Verification items for this drawing (mm, ordinates from the low corner). Give positions to 0.01 mm unless a question says otherwise; leave off trailing zeros. Loops run counter-clockwise (first coordinate to the right, second up) from the corner with the lowest first, then second, coordinate; pieces in that order, holes last. Notation, with made-up numbers: M 54,-29 L 103,-29 A9 ccw 103,-22 Z; hole C 72,-16 d6. An arc over 180 degrees is marked long. Put each result on its own line as item: value. Start each with the question number.
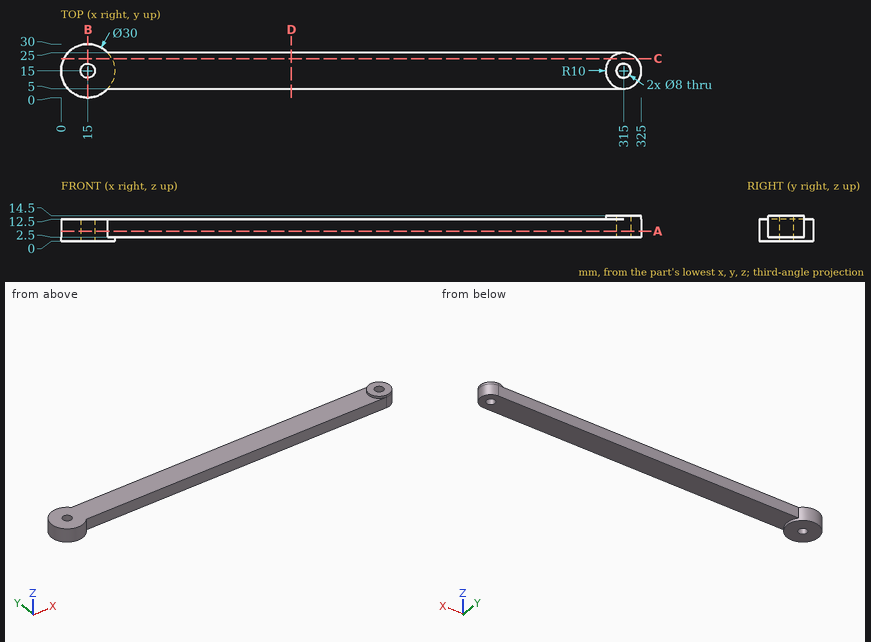
Q1. Go/stop test with flat-tipped pins: pin 1 (4 mm diameter, centred on x = 123, y = 26.5, fed in from +Z); pin 2 (16 mm diameter, centred on x = 227, y = 18, fed in from -Z); pin 3 (3 mm diameter, centred on y = 19.5, z = 10, fed in from -X); pin 4 (7 mm diameter, centred on x = 15, y = 15, fed in from -Z) (1 decimal). Record where each tip stops, or that it passes through.
Q2. Scan lines: L1, parallel to Y at x = 15, z = 4.75; L2, parallel to Y at x = 315, z = 5.5; L3, parallel to Y at x = 93, z = 9. Record each from-to range of solid material in increasing order.
Q3. Cross-section at C-C, the plane y = 21.75. Record the boundary of the cut face in (x, z), then the cut area to 3 significant figures.
Q4. Cross-section at A-A, the plane z = 5.75. Record the boundary of the cut face in (x, y), then the cut area to 3 significant figures.
Q5. Cross-section at B-B, the plane x = 15. Record the boundary of the cut face in (y, z), then the cut area to 3 significant figures.
Q6. Cross-section at D-D, the plane x = 129. Record the boundary of the cut face in (y, z), then the cut area to 3 significant figures.
Ans:
1. pin 1: stops at z = 12.5
1. pin 2: stops at z = 2.5
1. pin 3: stops at x = 0.3
1. pin 4: passes through
2. L1: y = 0 to 11, 19 to 30
2. L2: y = 5 to 11, 19 to 25
2. L3: y = 5 to 25
3. outline: M 1.6,0 L 28.4,0 L 28.4,2.5 L 322.38,2.5 L 322.38,14.5 L 307.62,14.5 L 307.62,12.5 L 1.6,12.5 Z
3. area: 3,300 mm^2
4. outline: M 26.18,5 L 315,5 A10 ccw 315,25 L 26.18,25 A15 ccw long Z; hole C 15,15 d8; hole C 315,15 d8
4. area: 6,490 mm^2
5. outline: M 0,0 L 11,0 L 11,12.5 L 0,12.5 Z; M 19,0 L 30,0 L 30,12.5 L 19,12.5 Z
5. area: 275 mm^2
6. outline: M 5,2.5 L 25,2.5 L 25,12.5 L 5,12.5 Z
6. area: 200 mm^2
